```python
from build123d import *

# Parameters (mm, degrees)
F0_R     = 22.733
F1_DEPTH = 1.5875


# Not quite as in the source:
# - a feature names something its author has since deleted; it is built from what else it names


with BuildPart() as f1:
    # F0 (on Front) → F1 (new body, symmetric)
    with BuildSketch(Plane.XZ):
        Polygon((22.3805892097, 23.3813975786), (-22.9507907903, 23.3813975786), (-36.3404007903, -23.6231935325), (35.7701992097, -23.6231935325), align=None)
        Circle(F0_R, mode=Mode.SUBTRACT)
    extrude(amount=F1_DEPTH, both=True)


solid = f1.part
```
The listing builds one solid part. Answer for the finished solid, in the listing's coordinates (mm). Coordinates: 2 decimals unless noted, no trailing zeros. Write each loop counter-clockwise with the first axis right and the second up, starting at its lowest first coordinate (ties: lowest second). Pieces come first, ordered by that corner, then holes. Notation, with made-up numbers: (85.5, 68.25) -> (94.5, 68.25) arc R8 ccw to (94.5, 74.25) -> close; hole circle Ø7 at (17.25, 54). An arc over 180 degrees is marked (long way). Write each question's results on one line, items separated by ' | '. Start each with the question number.
1) A cutting plane is placed at A-A (x = 0). Determine the outline of the cut face in (y, z), then the cut area to 3 significant figures.
2) A cutting plane is placed at C-C (y = 0.4). Determine the outline of the cut face in (x, z), then the cut area to 3 significant figures.
3) For a pull along X with two mould halves and no side action, classify faces 1 (the flat face through (-29.55, -0.02, 0.21)), 2 (the cylindrical face through (-4.9, 0, -22.2)), 3 (the flat face through (-11, -1.588, -21)) as +X half, -X half, draft (parallel to the pull), parting line (faces both ways), or undercut.
4) A cutting plane is placed at D-D (x = 28). Determine the outline of the cut face in (y, z).
5) A cutting plane is placed at B-B (z = 16). Determine the outline of the cut face in (x, y).
6) Straight lines are drawn through the part: probe 1 along Z at (x, y) = (0, 0.65); probe 2 along X at (y, z) = (-0.4, 10); probe 3 along X at (y, z) = (0.05, -17). For each, find the intervals that lie inside material, in ascending order.
7) A flat-ended cylindrical pin translates along its axis: pin 1 Ø1 at (y, z) = (-1, -18) entering from +X. Find the tip coordinate at first contact, or state that the pin passes through.
Values follow:
1) outline: (-1.59, -23.62) -> (1.59, -23.62) -> (1.59, -22.73) -> (-1.59, -22.73) -> close; (-1.59, 22.73) -> (1.59, 22.73) -> (1.59, 23.38) -> (-1.59, 23.38) -> close | area: 4.89 mm²
2) outline: (-36.34, -23.62) -> (35.77, -23.62) -> (22.38, 23.38) -> (-22.95, 23.38) -> close; hole circle Ø45.47 at (0, 0) | area: 1,140 mm²
3) face 1: -X half | face 2: undercut | face 3: draft
4) outline: (-1.59, -23.62) -> (1.59, -23.62) -> (1.59, 3.65) -> (-1.59, 3.65) -> close
5) outline: (-25.05, -1.59) -> (-16.15, -1.59) -> (-16.15, 1.59) -> (-25.05, 1.59) -> close; (16.15, -1.59) -> (24.48, -1.59) -> (24.48, 1.59) -> (16.15, 1.59) -> close
6) probe 1: -23.62 to -22.73, 22.73 to 23.38 | probe 2: -26.76 to -20.42, 20.42 to 26.19 | probe 3: -34.45 to -15.09, 15.09 to 33.88
7) pin 1: x = 34.31
